Input: dimensioned drawing with shaded views. Units: mm. Origin: part minimum x, y, z. Give positions to 0.01 mm unless a question says otherwise; leave off trailing zeros. Loops run counter-clockwise (first coordinate to the right, second up) from the corner with the lowest first, then second, coordinate; pieces in that order, holes last. Notation, with made-up numbers: (57, -35) -> (72, -35) arc R20 ccw to (72, -8) -> close; hole circle Ø2 at (9, 46). An arc over 180 degrees is marked (long way). Answer as a JSON object with one key per item and string values.
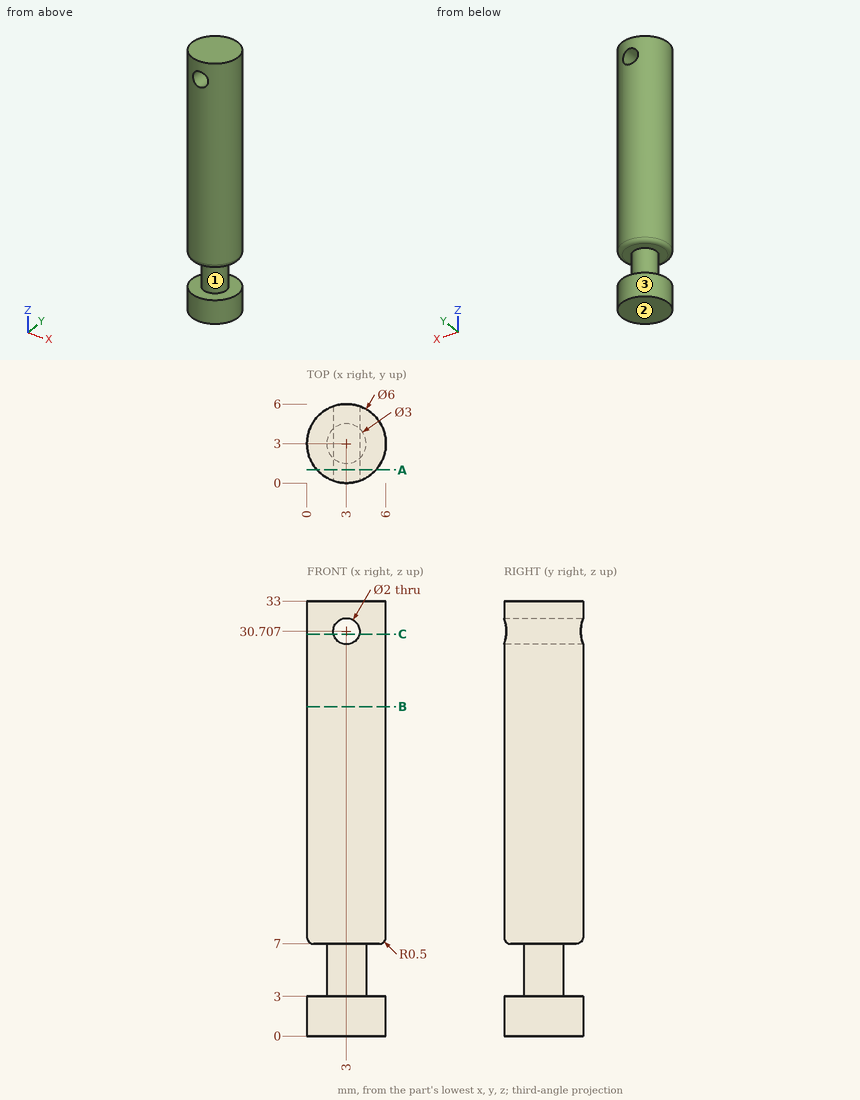
Q1. Draft query along Z for the marked faces 1, 2 and 3. Return one class per face: +Z half, -Z half, draft (parallel to the pull), parting line (faces both ways), or undercut.
Evaluation:
{"face 1": "undercut", "face 2": "-Z half", "face 3": "draft"}
Q2. Section A-A, the plane y = 1. Give the number of separate pieces and of enclosed holes in the cut face, then the cut area to 3 significant figures.
Evaluation:
{"separate pieces": "2", "enclosed holes": "1", "area": "126 mm2"}
Q3. Pin query (flat end, axial travel): pin 1 (2 mm diameter, centred on y = 1.5, z = 26.5, fed in from -X). Return the tip coordinate at first contact, or that it passes through.
Evaluation:
{"pin 1": "stops at x = 0.04"}
Q4. Section C-C, the plane z = 30.5. Return the cut outline in (x, y).
Evaluation:
{"outline": "(2.02, 0.16) -> (2.02, 5.84) arc R3 ccw to start; (3.98, 0.16) arc R3 ccw to (3.98, 5.84) -> close"}
Q5. Section B-B, the plane z = 25. Return the cut outline in (x, y), then the cut area to 3 significant figures.
Evaluation:
{"outline": "circle Ø6 at (3, 3)", "area": "28.3 mm2"}
Q6. Ray query, line 1 along Z through (x, y) = (5.25, 1.75) (1 decimal); line 2 along Z through (x, y) = (2.25, 5) (1 decimal); line 3 along Z through (x, y) = (3.5, 2.5). Return the intervals inside material, ascending.
Evaluation:
{"line 1": "z = 0 to 3, 7 to 33", "line 2": "z = 0 to 3, 7 to 30, 31.4 to 33", "line 3": "z = 0 to 29.84, 31.57 to 33"}
